Print and shaded views of the part. All mm, measured from the part's lowest x, y and z. A direction names the side the tool comes from. Round coordinates to 2 decimals unless told otherwise and drop trailing zeros. Write each loop counter-clockwise with the first axis right and the second up, starting at its lowest first coordinate (ties: lowest second). Pieces come first, ordered by that corner, then holes. Notation, with made-up numbers: (16, 89) - (35, 89) arc R10 cw to (35, 106) - close; hole circle Ø7 at (26, 69.5). An arc over 180 degrees is marked (long way). One line per item, written item: value.
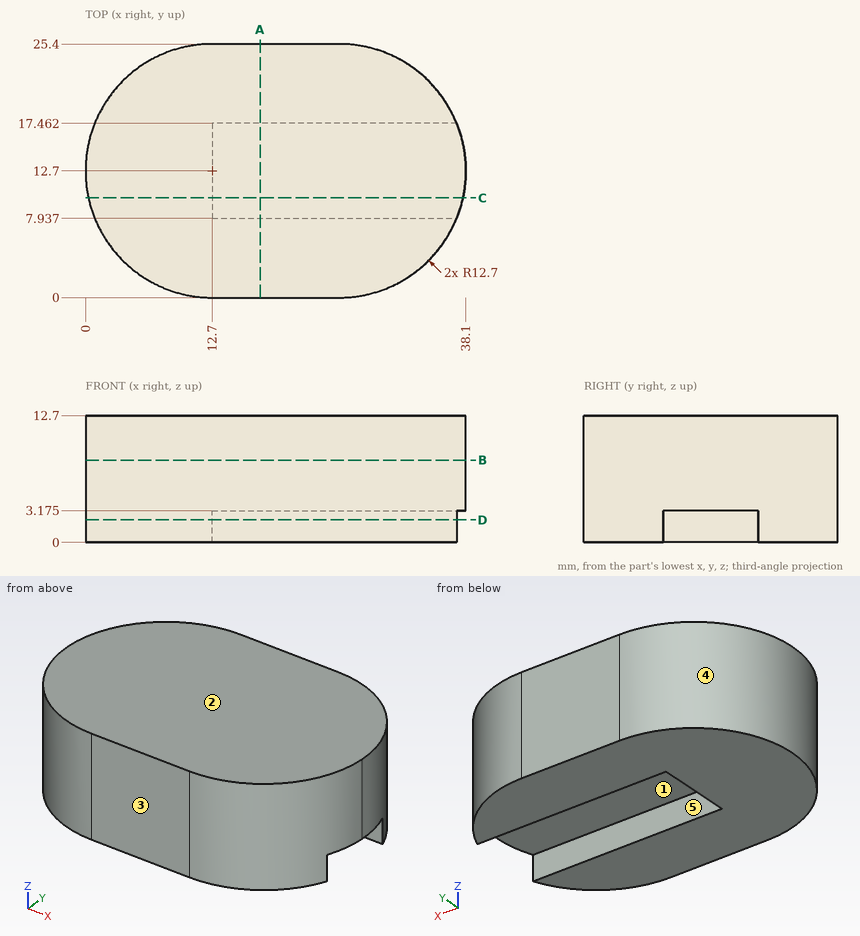
1. Band-saw the part on A-A on x = 17.5. Write the cut outline in (y, z) (1 decimal).
Report:
outline: (0, 0) - (7.9, 0) - (7.9, 3.2) - (17.5, 3.2) - (17.5, 0) - (25.4, 0) - (25.4, 12.7) - (0, 12.7) - close
2. Band-saw the part on D-D on z = 2.25. Write the cut outline in (x, y).
Report:
outline: (12.7, 0) - (25.4, 0) arc R12.7 ccw to (37.17, 7.94) - (12.7, 7.94) - (12.7, 17.46) - (37.17, 17.46) arc R12.7 ccw to (25.4, 25.4) - (12.7, 25.4) arc R12.7 ccw to start
3. Band-saw the part on B-B on z = 8.25. Write the cut outline in (x, y), plus the area to 3 significant figures.
Report:
outline: (12.7, 0) - (25.4, 0) arc R12.7 ccw to (25.4, 25.4) - (12.7, 25.4) arc R12.7 ccw to start
area: 829 mm²
4. Wall check: probe 1 along Z at (x, y) = (14, 15.5) (1 decimal); probe 2 along X at (y, z) = (16.25, 7.25) (1 decimal); probe 3 along X at (y, z) = (6, 9.5). Give the ranges that are in metal, low to high. Write a range as [from, to].
Report:
probe 1: [3.2, 12.7]
probe 2: [0.5, 37.6]
probe 3: [1.91, 36.19]
5. Drop flat-ended pins along their axis: pin 1 (5 mm diameter, centred on y = 22.5, z = 5, fed in from -X); pin 2 (2.5 mm diameter, centred on y = 13, z = 1, fed in from +X); pin 3 (2.5 mm diameter, centred on x = 30.5, z = 1.5, fed in from +Y). Give the stop position or say it passes through.
Report:
pin 1: x = 2.31
pin 2: x = 12.7
pin 3: y = 24.8
6. Band-saw the part on C-C on y = 10. Write the cut outline in (x, z) (1 decimal).
Report:
outline: (0.3, 0) - (12.7, 0) - (12.7, 3.2) - (37.8, 3.2) - (37.8, 12.7) - (0.3, 12.7) - close
7. Tool access for the marked faces 4 and 5: list every direction of +Z, -Z, +X, -X, +Y, -Y with a clear straight run to the whole face (end or side of a thin tool).
Report:
face 4: +Z, -Z, -X
face 5: -Z, +X
8. Mould opens along Y. For the marked faces 1, 2 and 3 say: released by +Y, released by -Y, zero draft, split by the parting line, or undercut.
Report:
face 1: undercut
face 2: zero draft
face 3: released by -Y
